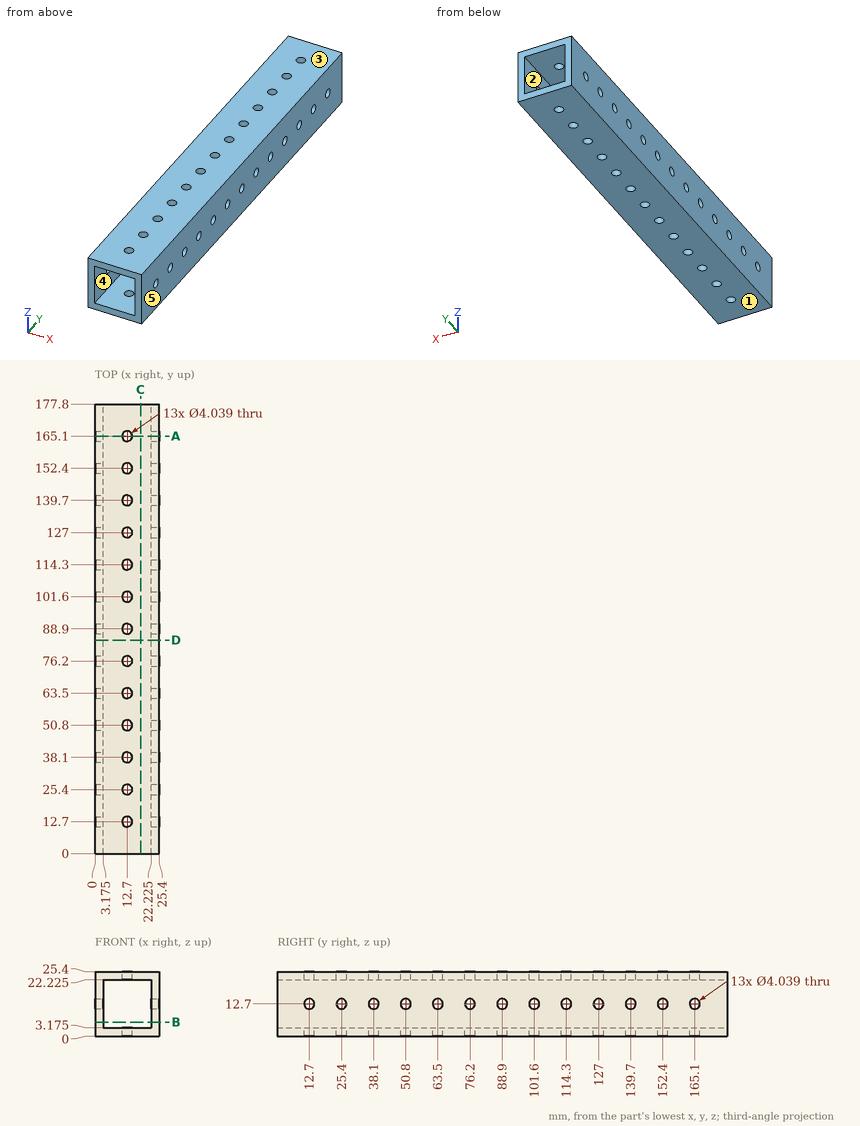
The drawing under review shows one solid part. Ordinate dimensions are in mm from its lowest x, y, z. A direction names the side the tool comes from. Coordinates: 2 decimals unless noted, no trailing zeros. Write each loop counter-clockwise with the first axis right and the second up, starting at its lowest first coordinate (ties: lowest second). Pieces come first, ordered by that corner, then holes. Notation, with made-up numbers: (-2.75, 70.25) - (14.25, 70.25) arc R28 ccw to (14.25, 103.25) - close; hole circle Ø7 at (-38.75, 57). An arc over 180 degrees is marked (long way). Put each result on its own line as item: value.
1. Add section C-C, the plane x = 18. Give the boundary of the cut face in (y, z) (1 decimal), then the cut area to 3 significant figures.
Values found:
outline: (0, 0) - (177.8, 0) - (177.8, 3.2) - (0, 3.2) - close; (0, 22.2) - (177.8, 22.2) - (177.8, 25.4) - (0, 25.4) - close
area: 1,130 mm²
2. Mouldability with a two-part tool opening along Z and no side actions: class the marked faces 3, 4 and 5 as released by +Z, released by -Z, zero draft, split by the parting line, or undercut.
Values found:
face 3: released by +Z
face 4: undercut
face 5: zero draft
3. Wall thickness on probe 1 along X at (y, z) = (59, 12.5) (1 decimal); probe 2 along X at (y, z) = (90, 23.5) (1 decimal): over which ranges is each line inside the solid? List them lowest first.
Values found:
probe 1: 0 to 3.2, 22.2 to 25.4
probe 2: 0 to 11, 14.4 to 25.4
4. Machinability: for the marked faces 1 and 2, which of the approach directions +Z, -Z, +X, -X, +Y, -Y give a long, thin tool a straight path to every point of the face, cutting with its end or side? Answer none if there is none.
Values found:
face 1: -Z, +X, -X, +Y, -Y
face 2: +Y, -Y
5. Add section A-A, the plane y = 165.1. Give the boundary of the cut face in (x, z) (1 decimal), then the cut area to 3 significant figures.
Values found:
outline: (0, 0) - (10.7, 0) - (10.7, 3.2) - (3.2, 3.2) - (3.2, 10.7) - (0, 10.7) - close; (0, 14.7) - (3.2, 14.7) - (3.2, 22.2) - (10.7, 22.2) - (10.7, 25.4) - (0, 25.4) - close; (14.7, 0) - (25.4, 0) - (25.4, 10.7) - (22.2, 10.7) - (22.2, 3.2) - (14.7, 3.2) - close; (14.7, 22.2) - (22.2, 22.2) - (22.2, 14.7) - (25.4, 14.7) - (25.4, 25.4) - (14.7, 25.4) - close
area: 231 mm²
6. Add section D-D, the plane y = 84.5. Give the boundary of the cut face in (x, z) (1 decimal), then the cut area to 3 significant figures.
Values found:
outline: (0, 0) - (25.4, 0) - (25.4, 25.4) - (0, 25.4) - close; hole (3.2, 3.2) - (22.2, 3.2) - (22.2, 22.2) - (3.2, 22.2) - close
area: 282 mm²
7. Add section B-B, the plane z = 5.5. Give the boundary of the cut face in (x, y) (1 decimal), then the cut area to 3 significant figures.
Values found:
outline: (0, 0) - (3.2, 0) - (3.2, 177.8) - (0, 177.8) - close; (22.2, 0) - (25.4, 0) - (25.4, 177.8) - (22.2, 177.8) - close
area: 1,130 mm²
8. For pin 1 (2.5 mm diameter, centred on y = 50.8, z = 12.7, fed in from +X), flat-tipped, find the tip position at first contact; note if it passes through.
Values found:
pin 1: through
